Model file for the job. Use its own axes, mm. Round coordinates to 2 decimals unless told otherwise and drop trailing zeros. Order: outer loops, then holes, each group sorted by start corner. A loop starts at its lowest first (then second) coordinate and runs counter-clockwise, first axis right, second up. Notation, with made-up numbers: (-7.75, 89.5) -> (11.25, 89.5) arc R22 cw to (11.25, 126.5) -> close; hole circle Ø5 at (1.25, 66). An arc over 180 degrees is marked (long way). Put each result on its own line as item: value. Start each with the question number.
Q1. Pull direction X, two halves, no side cores. Call faces 1 (the face through (-7.79, 10.17, 1.57)), 2 (the face through (0, 0, 3.175)), 3 (the face through (-67.9, -66.73, 1.57)): released by +X, released by -X, zero draft, split by the parting line, or undercut.
Q2. Cut at A-A, the plane x = 65.5. List the corners of the cut face in (y, z) (3 decimals), and give its area (3 significant figures).
Q3. Probe L1, parallel to X at y = -64.5, z = 2.45; L2, parallel to Y at x = -33, z = 0.5; L3, parallel to Y at x = -61, z = 1.35. List the from-to ranges inside material, lowest first.
Q4. Cut at D-D, the plane x = -80. List the corners of the cut face in (y, z) (3 decimals).
Q5. Flat gauge pins, fed straight in: P1, Ø8, axis at x = -69.5, y = -56, coming from the -Z side; P2, Ø1, axis at x = -27, z = 2, coming from the -Y side; P3, Ø1.5, axis at x = -35, z = 1, coming from the +Y side. Where does each tip first touch, or does it go through?
Q6. Cut at B-B, the plane z = 1.25. List the corners of the cut face in (x, y).
Q7. Cut at C-C, the plane y = -79. List the corners of the cut face in (x, z) (3 decimals).
from build123d import *

# Parameters (mm, degrees)
F0_R     = 6.35
F1_DEPTH = 3.175


with BuildPart() as f1:
    # F0 (on Top) → F1 (new body)
    with BuildSketch(Plane.XY):
        with BuildLine():
            Line((76.332177, 94.292689), (-8.980256, 8.980256))
            Line((-8.980256, 8.980256), (-94.292689, -76.332177))
            ThreePointArc((-94.292689, -76.332177), (-96.152561, -80.822305), (-94.292689, -85.312433))
            Line((-94.292689, -85.312433), (-89.802561, -89.802561))
            Line((-89.802561, -89.802561), (-85.312433, -94.292689))
            ThreePointArc((-85.312433, -94.292689), (-80.822305, -96.152561), (-76.332177, -94.292689))
            Line((-76.332177, -94.292689), (8.980256, -8.980256))
            Line((8.980256, -8.980256), (94.292689, 76.332177))
            ThreePointArc((94.292689, 76.332177), (96.152561, 80.822305), (94.292689, 85.312433))
            Line((94.292689, 85.312433), (89.802561, 89.802561))
            Line((89.802561, 89.802561), (85.312433, 94.292689))
            ThreePointArc((85.312433, 94.292689), (80.822305, 96.152561), (76.332177, 94.292689))
        make_face()
        with Locations((-62.861793, -62.861793)):
            Circle(F0_R, mode=Mode.SUBTRACT)
        with Locations((-30.083858, -30.083858)):
            Circle(F0_R, mode=Mode.SUBTRACT)
        with Locations((30.083858, 30.083858)):
            Circle(F0_R, mode=Mode.SUBTRACT)
        with Locations((62.861793, 62.861793)):
            Circle(F0_R, mode=Mode.SUBTRACT)
    extrude(amount=F1_DEPTH)


solid = f1.part
Ans:
1. face 1: released by -X
1. face 2: zero draft
1. face 3: undercut
2. outline: (47.539, 0) -> (57.086, 0) -> (57.086, 3.175) -> (47.539, 3.175) -> close; (68.638, 0) -> (83.461, 0) -> (83.461, 3.175) -> (68.638, 3.175) -> close
2. area: 77.4 mm^2
3. L1: x = -82.46 to -69, -56.73 to -46.54
3. L2: y = -50.96 to -35.72, -24.44 to -15.04
3. L3: y = -78.96 to -68.93, -56.79 to -43.04
4. outline: (-96.099, 0) -> (-62.039, 0) -> (-62.039, 3.175) -> (-96.099, 3.175) -> close
5. P1: stops at z = 0
5. P2: stops at y = -45.46
5. P3: stops at y = -16.29
6. outline: (-94.29, -85.31) -> (-85.31, -94.29) arc R6.35 ccw to (-76.33, -94.29) -> (94.29, 76.33) arc R6.35 ccw to (94.29, 85.31) -> (85.31, 94.29) arc R6.35 ccw to (76.33, 94.29) -> (-94.29, -76.33) arc R6.35 ccw to start; hole circle Ø12.7 at (-62.86, -62.86); hole circle Ø12.7 at (-30.08, -30.08); hole circle Ø12.7 at (30.08, 30.08); hole circle Ø12.7 at (62.86, 62.86)
7. outline: (-95.885, 0) -> (-61.039, 0) -> (-61.039, 3.175) -> (-95.885, 3.175) -> close
